Can you work these out from the model? Positions are in its coordinate system, mm. Coordinates: 2 decimals unless noted, no trailing zeros. Order: outer loops, then holes, each group sorted by start corner. A loop starts at its lowest first (then second) coordinate and runs counter-clockwise, first axis right, second up. Notation, with made-up numbers: (48.5, -33.75) -> (84.5, -33.75) arc R9 cw to (84.5, -25.75) -> close; hole circle Ø11 at (71.25, -28.75). An arc over 180 degrees is marked (long way). Return JSON: item names as keys, results as strings. Group by question number.
1) If we section it at A-A, the plane z = 5: Please give me the cut outline in (x, y).
2) Thinking about a two-plate mould opening in Z: for faces 1 (the cylindrical face through (-53.1, -13.46, 13.14)), 2 (the cylindrical face through (-53.1, -13.46, 0.86)), 3 (the flat face through (-45, -16, 7)), 4 (the cylindrical face through (-51.71, -13.54, 5.38)), which applies, +Z half, -Z half, draft (parallel to the pull), parting line (faces both ways), or undercut?
3) If we section it at B-B, the plane x = -50: Please give me the cut outline in (y, z).
4) If we section it at D-D, the plane y = -13.2: Please give me the cut outline in (x, z), then the cut area to 3 significant figures.
5) If I drill on probe 1 along Z at (x, y) = (-51.5, -14.2); probe 2 along X at (y, z) = (-13.45, 5); probe 3 along Z at (x, y) = (-49.75, -13), over which ranges is the centre line in solid material (lowest first)? Write a range as from..to.
6) If we section it at C-C, the plane y = -14.7: Please give me the cut outline in (x, z), then the cut area to 3 significant figures.
from build123d import *
from build123d.topology import SkipClean

# Parameters (mm, degrees)
SKETCH1_R                      = 40
SKETCH1_R_2                    = 38
BOSS_EXTRUDE1_DEPTH            = 200
SKETCH2_R                      = 40
BOSS_EXTRUDE2_DEPTH            = 2
BOSS_EXTRUDE3_DEPTH            = 107
BOSS_EXTRUDE4_DEPTH            = 2
SKETCH5_R                      = 1.75
CUT_EXTRUDE1_DEPTH             = 225.428162226
CUT_EXTRUDE2_REACH             = 218.296
SKETCH6_R                      = 4
CUT_EXTRUDE2_DIRECTION_2_REACH = 218.296
CIRPATTERN1_COUNT              = 2
CIRPATTERN1_ANGLE              = 90
BOSS_EXTRUDE5_REACH            = 241.742
BOSS_EXTRUDE5_END_RADIUS       = 40
SKETCH7_W                      = 14
SKETCH7_H                      = 5
CUT_EXTRUDE3_REACH             = 221.818
SKETCH8_R                      = 1.75
FILLET1_R                      = 3
CUT_EXTRUDE4_REACH             = 220.598
SKETCH9_R                      = 0.25
BOSS_EXTRUDE6_START            = 2
BOSS_EXTRUDE6_DEPTH            = 2
CUT_EXTRUDE5_REACH             = 220.147


with BuildPart() as part:
    # Sketch1 → Boss-Extrude1 (new body)
    with BuildSketch(Plane.XY):
        Circle(SKETCH1_R)
        Circle(SKETCH1_R_2, mode=Mode.SUBTRACT)
    extrude(amount=BOSS_EXTRUDE1_DEPTH)

    # Sketch2 → Boss-Extrude2 (add)
    with BuildSketch(Plane.XY.offset(180)):
        Circle(SKETCH2_R)
    extrude(amount=BOSS_EXTRUDE2_DEPTH)

    # Sketch3 → Boss-Extrude3 (add)
    with BuildSketch(Plane(origin=(0, 0, 0), x_dir=(-1, 0, 0), z_dir=(0, 0, -1))):
        with BuildLine():
            Line((-24, -32), (-72, -32))
            Line((-72, -32), (-72, -30))
            Line((-72, -30), (-26.457513111, -30))
            ThreePointArc((-26.457513111, -30), (-25.248567431, -31.024342744), (-24, -32))
        make_face()
        with BuildLine():
            Line((-24, 32), (-72, 32))
            Line((-72, 32), (-72, 30))
            Line((-72, 30), (-26.457513111, 30))
            ThreePointArc((-26.457513111, 30), (-25.248567431, 31.024342744), (-24, 32))
        make_face()
    extrude(amount=-BOSS_EXTRUDE3_DEPTH)

    # Sketch4 → Boss-Extrude4 (add)
    with BuildSketch(Plane.XY.offset(107)):
        with BuildLine():
            Line((72, -32), (24, -32))
            ThreePointArc((24, -32), (40, 0), (24, 32))
            Line((24, 32), (72, 32))
            Line((72, 32), (72, -32))
        make_face()
    extrude(amount=BOSS_EXTRUDE4_DEPTH)

    # Sketch5 → Cut-Extrude1 (cut, through all)
    with BuildSketch(Plane(origin=(0, 32, 0), x_dir=(1, 0, 0), z_dir=(0, 1, 0))):
        with Locations(Location((43.5, -102.5, 0), (0, 0, 270))):
            Circle(SKETCH5_R)
        with Locations(Location((43.5, -3.5, 0), (0, 0, 270))):
            Circle(SKETCH5_R)
        with Locations(Location((68.5, -78, 0), (0, 0, 270))):
            Circle(SKETCH5_R)
    extrude(amount=-CUT_EXTRUDE1_DEPTH, mode=Mode.SUBTRACT)

    # Sketch6 → Cut-Extrude2 (cut, up to next)
    with BuildSketch(Plane(origin=(0, 0, 0), x_dir=(0, 0, 1), z_dir=(-0.7071067811865488, 0.7071067811865464, 0)), mode=Mode.PRIVATE) as cut_extrude2_sk1:
        with Locations(Location((187, 0, 0), (0, 0, 90))):
            Circle(SKETCH6_R)
    cut_extrude2_tool1 = extrude(cut_extrude2_sk1.sketch, amount=-CUT_EXTRUDE2_REACH, mode=Mode.PRIVATE) & part.part
    cut_extrude2 = cut_extrude2_tool1.solids().sort_by_distance((0, 0, 187))[0]
    add(cut_extrude2, mode=Mode.SUBTRACT)

    # Sketch6 → Cut-Extrude2 direction 2 (cut, up to next)
    with BuildSketch(Plane(origin=(0, 0, 0), x_dir=(0, 0, 1), z_dir=(-0.7071067811865488, 0.7071067811865464, 0)), mode=Mode.PRIVATE) as cut_extrude2_direction_2_sk1:
        with Locations(Location((187, 0, 0), (0, 0, 90))):
            Circle(SKETCH6_R)
    cut_extrude2_direction_2_tool1 = extrude(cut_extrude2_direction_2_sk1.sketch, amount=CUT_EXTRUDE2_DIRECTION_2_REACH, mode=Mode.PRIVATE) & part.part
    cut_extrude2_direction_2 = cut_extrude2_direction_2_tool1.solids().sort_by_distance((0, 0, 187))[0]
    add(cut_extrude2_direction_2, mode=Mode.SUBTRACT)

    # CirPattern1: Cut-Extrude2, Cut-Extrude2 direction 2 ×2 about axis
    cirpattern1_axis = Axis((0, 0, -0.7), (0, 0, 1))
    add([cut_extrude2.rotate(cirpattern1_axis, i * CIRPATTERN1_ANGLE / (CIRPATTERN1_COUNT - 1)) for i in range(1, CIRPATTERN1_COUNT)], mode=Mode.SUBTRACT)
    add([cut_extrude2_direction_2.rotate(cirpattern1_axis, i * CIRPATTERN1_ANGLE / (CIRPATTERN1_COUNT - 1)) for i in range(1, CIRPATTERN1_COUNT)], mode=Mode.SUBTRACT)

    # Boss-Extrude5: up to this cylinder (the profile starts outside it)
    boss_extrude5_end = Plane(origin=(0, 0, 7), z_dir=(0, 0, -1)) * Cylinder(BOSS_EXTRUDE5_END_RADIUS, 564.484, mode=Mode.PRIVATE)
    # Sketch7 → Boss-Extrude5 (add, up to the surface)
    with BuildSketch(Plane(origin=(-54, 0, 0), x_dir=(0, 0, -1), z_dir=(1, 0, 0)), mode=Mode.PRIVATE) as boss_extrude5_sk1:
        with Locations((-7, -13.5)):
            Rectangle(SKETCH7_W, SKETCH7_H)
    boss_extrude5_tool1 = extrude(boss_extrude5_sk1.sketch, amount=BOSS_EXTRUDE5_REACH, mode=Mode.PRIVATE) - boss_extrude5_end
    add(boss_extrude5_tool1.solids().sort_by_distance((-54, -13.5, 7))[0])
    # Sketch7 → Boss-Extrude5 (add, up to the surface)
    with BuildSketch(Plane(origin=(-54, 0, 0), x_dir=(0, 0, -1), z_dir=(1, 0, 0)), mode=Mode.PRIVATE) as boss_extrude5_sk2:
        with Locations((-7, 13.5)):
            Rectangle(SKETCH7_W, SKETCH7_H)
    boss_extrude5_tool2 = extrude(boss_extrude5_sk2.sketch, amount=BOSS_EXTRUDE5_REACH, mode=Mode.PRIVATE) - boss_extrude5_end
    add(boss_extrude5_tool2.solids().sort_by_distance((-54, 13.5, 7))[0])

    # Cut-Extrude3: up to this face of the body (flat: up to its plane)
    cut_extrude3_end = Plane(part.part.faces().sort_by_distance((-45.33030278, 16, 7))[0])
    # Sketch8 → Cut-Extrude3 (cut, up to the picked face)
    with BuildSketch(Plane.XZ.offset(16), mode=Mode.PRIVATE) as cut_extrude3_sk1:
        with Locations(Location((-50, 5, 0), (0, 0, 270))):
            Circle(SKETCH8_R)
    cut_extrude3_tool1 = split(extrude(cut_extrude3_sk1.sketch, amount=-CUT_EXTRUDE3_REACH, mode=Mode.PRIVATE), bisect_by=cut_extrude3_end, keep=Keep.BOTH, mode=Mode.PRIVATE)
    add(cut_extrude3_tool1.solids().sort_by(Axis((-50, -16, 5), (0, 1, 0)))[0], mode=Mode.SUBTRACT)

    # Fillet1
    fillet1_edges = [part.edges().sort_by_distance(p)[0] for p in [
        (-54, -13.5, 14),
        (-54, -13.5, 0),
        (-54, 13.5, 0),
        (-54, 13.5, 14),
    ]]
    fillet(fillet1_edges, radius=FILLET1_R)

    # Sketch9 → Cut-Extrude4 (cut, up to next)
    with BuildSketch(Plane.XZ.offset(-11), mode=Mode.PRIVATE) as cut_extrude4_sk1:
        with Locations(Location((-44, 7, 0), (0, 0, 270))):
            Circle(SKETCH9_R)
    cut_extrude4_tool1 = extrude(cut_extrude4_sk1.sketch, amount=-CUT_EXTRUDE4_REACH, mode=Mode.PRIVATE) & part.part
    add(cut_extrude4_tool1.solids().sort_by_distance((-44, 11, 7))[0], mode=Mode.SUBTRACT)

    # Sketch10 → Boss-Extrude6 (add)
    with SkipClean():  # the faces are left unmerged after this step: merging them gives an invalid solid
        with BuildSketch(Plane(origin=(0, 0, 0), x_dir=(-1, 0, 0), z_dir=(0, 0, -1)).offset(BOSS_EXTRUDE6_START)):
            with BuildLine():
                ThreePointArc((10, -36.66060556), (0, -38), (-10, -36.66060556))
                Line((-10, -36.66060556), (-10, -38.729833462))
                ThreePointArc((-10, -38.729833462), (0, -40), (10, -38.729833462))
                Line((10, -38.729833462), (10, -36.66060556))
            make_face()
            with BuildLine():
                ThreePointArc((10, 38.729833462), (0, 40), (-10, 38.729833462))
                Line((-10, 38.729833462), (-10, 36.66060556))
                ThreePointArc((-10, 36.66060556), (0, 38), (10, 36.66060556))
                Line((10, 36.66060556), (10, 38.729833462))
            make_face()
        extrude(amount=-BOSS_EXTRUDE6_DEPTH)

    # Sketch11 → Cut-Extrude5 (cut, up to next)
    with BuildSketch(Plane.XY.offset(200), mode=Mode.PRIVATE) as cut_extrude5_sk1:
        with BuildLine():
            ThreePointArc((-39.953981252, 1.918171548), (-25.55703566, -30.770731683), (9.219033253, -38.923121996))
            ThreePointArc((9.219033253, -38.923121996), (103.998908328, 0), (9.219033253, 38.923121996))
            ThreePointArc((9.219033253, 38.923121996), (4.476281437, 39.748747207), (-0.331307503, 39.998627918))
            ThreePointArc((-0.331307503, 39.998627918), (-96.996927129, 100.925197981), (-39.953981252, 1.918171548))
        make_face()
    cut_extrude5_tool1 = extrude(cut_extrude5_sk1.sketch, amount=-CUT_EXTRUDE5_REACH, mode=Mode.PRIVATE) & part.part
    add(cut_extrude5_tool1.solids().sort_by_distance((-7.679141, 27.95673, 200))[0], mode=Mode.SUBTRACT)


solid = part.part
Result sheet:
{
 "1": {"outline": "(-54, -16) -> (-51.75, -16) -> (-51.75, -11) -> (-54, -11) -> close; (-48.25, -16) -> (-36.66, -16) arc R40 cw to (-38.46, -11) -> (-48.25, -11) -> close"},
 "2": {"face 1": "+Z half", "face 2": "-Z half", "face 3": "draft", "face 4": "undercut"},
 "3": {"outline": "(-16, 0) -> (-11, 0) -> (-11, 3.25) -> (-16, 3.25) -> close; (-16, 6.75) -> (-11, 6.75) -> (-11, 14) -> (-16, 14) -> close"},
 "4": {"outline": "(-54, 3) arc R3 ccw to (-51, 0) -> (-37.76, 0) -> (-37.76, 14) -> (-51, 14) arc R3 ccw to (-54, 11) -> close; hole circle Ø3.5 at (-50, 5)", "area": "214 mm2"},
 "5": {"probe 1": "z = 0.04..4.1, 5.9..13.96", "probe 2": "x = -54..-51.75, -48.25..-37.67", "probe 3": "z = 0..3.27, 6.73..14"},
 "6": {"outline": "(-54, 3) arc R3 ccw to (-51, 0) -> (-37.2, 0) -> (-37.2, 14) -> (-51, 14) arc R3 ccw to (-54, 11) -> close; hole circle Ø3.5 at (-50, 5)", "area": "222 mm2"}
}
